The model under review builds one solid part; all positions refer to its coordinate system, in mm. A direction names the side the tool comes from. Coordinates: 2 decimals unless noted, no trailing zeros. Write each loop counter-clockwise with the first axis right and the second up, starting at its lowest first coordinate (ties: lowest second). Pieces come first, ordered by that corner, then holes.
1) Add section B-B, the plane x = 3. State the section outline as (y, z) points.
2) For P1, Ø1, axis at x = 7.5, y = -1.5, coming from the -Z side; P2, Ø4, axis at x = 22.5, z = -5, coming from the +Y side; P3, Ø0.6, axis at y = -1, z = -16, coming from the -X side, all flat-tipped, find the tip position at first contact; note any pin that passes through.
3) Add section A-A, the plane z = -14.5. State the section outline as (x, y) points, then the cut area to 3 significant figures.
4) Add section C-C, the plane y = 4.5. State the section outline as (x, z) points.
5) For line 1 (Y direction, x = 6, z = -8.75); line 2 (Y direction, x = 30.5, z = -13.5), list the stretches that pass through material, from the lowest coordinate up.
6) Add section D-D, the plane x = 28.5. State the section outline as (y, z) points.
7) Mouldability with a two-part tool opening along Z and no side actions: class faces 1 (the cylindrical face through (25.463, 8.951, -8.033)), 2 (the cylindrical face through (9.513, 0.507, -0.911)), 3 (the flat face through (16, 1, -13)) as released by +Z, released by -Z, zero draft, split by the parting line, or undercut.
8) Machinability: for faces 4 (the flat face through (13, -1, -22.429)), 5 (the flat face through (0.278, -1, -13)), 6 (the cylindrical face through (0.688, 0.507, -21.893)), which of the approach directions +Z, -Z, +X, -X, +Y, -Y give a long, thin tool a straight path to every point of the face, cutting with its end or side? Answer none if there is none.
from build123d import *

# Parameters (mm, degrees)
SKETCH1_W           = 33
SKETCH1_H           = 25
BOSS_EXTRUDE1_DEPTH = 1
CUT_EXTRUDE1_DEPTH  = 2
SKETCH3_R           = 0.4
SKETCH3_R_2         = 0.442084783
SKETCH3_R_3         = 0.458227678
CUT_EXTRUDE2_DEPTH  = 2
SKETCH4_R           = 0.75
BOSS_EXTRUDE2_DEPTH = 17
BOSS_EXTRUDE3_DEPTH = 2


with BuildPart() as part:
    # Sketch1 → Boss-Extrude1 (new body)
    with BuildSketch(Plane(origin=(0, 0, 0), x_dir=(1, 0, 0), z_dir=(0, 1, 0))):
        with Locations((16.5, 12.5)):
            Rectangle(SKETCH1_W, SKETCH1_H)
    extrude(amount=BOSS_EXTRUDE1_DEPTH)

    # Sketch2 → Cut-Extrude1 (cut, through all)
    with BuildSketch(Plane.XZ):
        Polygon((33, 0), (26.482981269, 0), (33, -7.837809095), align=None)
        Polygon((33, -17.162190905), (33, -25), (26.482981269, -25), align=None)
    extrude(amount=-CUT_EXTRUDE1_DEPTH, mode=Mode.SUBTRACT)

    # Sketch3 → Cut-Extrude2 (cut, through all)
    with BuildSketch(Plane(origin=(0, 1, 0), x_dir=(1, 0, 0), z_dir=(0, 1, 0))):
        with Locations((7.143852183, 23.936106005)):
            Circle(SKETCH3_R)
        with Locations((9.143852183, 23.936106005)):
            Circle(SKETCH3_R)
        with Locations((11.143852183, 23.936106005)):
            Circle(SKETCH3_R)
        with Locations((13.143852183, 23.936106005)):
            Circle(SKETCH3_R)
        with Locations((15.143852183, 23.936106005)):
            Circle(SKETCH3_R)
        with Locations((17.143852183, 23.936106005)):
            Circle(SKETCH3_R)
        with Locations((19.143852183, 23.936106005)):
            Circle(SKETCH3_R)
        with Locations((21.143852183, 23.936106005)):
            Circle(SKETCH3_R)
        with Locations((23.143852183, 23.936106005)):
            Circle(SKETCH3_R)
        with Locations((25.143852183, 23.936106005)):
            Circle(SKETCH3_R)
        with Locations((25.143852183, 1.063893995)):
            Circle(SKETCH3_R)
        with Locations((23.143852183, 1.063893995)):
            Circle(SKETCH3_R)
        with Locations((21.143852183, 1.063893995)):
            Circle(SKETCH3_R)
        with Locations((19.143852183, 1.063893995)):
            Circle(SKETCH3_R)
        with Locations((17.143852183, 1.063893995)):
            Circle(SKETCH3_R)
        with Locations((15.143852183, 1.063893995)):
            Circle(SKETCH3_R)
        with Locations((13.143852183, 1.063893995)):
            Circle(SKETCH3_R)
        with Locations((11.143852183, 1.063893995)):
            Circle(SKETCH3_R)
        with Locations((9.143852183, 1.063893995)):
            Circle(SKETCH3_R)
        with Locations((7.143852183, 1.063893995)):
            Circle(SKETCH3_R)
        with Locations((0.784299075, 22.325061426)):
            Circle(SKETCH3_R_2)
        with Locations((24.152709784, 2.722277331)):
            Circle(SKETCH3_R_3)
    extrude(amount=-CUT_EXTRUDE2_DEPTH, mode=Mode.SUBTRACT)

    # Sketch4 → Boss-Extrude2 (add)
    with BuildSketch(Plane(origin=(0, 1, 0), x_dir=(1, 0, 0), z_dir=(0, 1, 0))):
        with Locations((26.211922043, 8)):
            Circle(SKETCH4_R)
    extrude(amount=BOSS_EXTRUDE2_DEPTH)

    # Sketch5 → Revolve1 (revolve)
    with BuildSketch(Plane.XY.offset(-8)):
        with BuildLine():
            Line((26.211922043, 18), (26.211922043, 23))
            ThreePointArc((26.211922043, 23), (25.525593233, 22.727999503), (25.211922043, 22.059686783))
            Line((25.211922043, 22.059686783), (24.961922043, 18))
            ThreePointArc((24.961922043, 18), (25.081321038, 17.489279713), (25.461922043, 17.128399944))
            Line((25.461922043, 17.128399944), (25.461922043, 18))
            Line((25.461922043, 18), (26.211922043, 18))
        make_face()
    revolve(axis=Axis((26.211922043, 18, -8), (0, 1, 0)))

    # Sketch6 → Boss-Extrude3 (add)
    with BuildSketch(Plane.XZ):
        with BuildLine():
            Line((24.507853381, -22.428957603), (0.778175079, -22.428957603))
            ThreePointArc((0.778175079, -22.428957603), (0.424621688, -22.282510994), (0.278175079, -21.928957603))
            Line((0.278175079, -21.928957603), (0.278175079, -2.903294195))
            ThreePointArc((0.278175079, -2.903294195), (0.424621688, -2.549740805), (0.778175079, -2.403294195))
            Line((0.778175079, -2.403294195), (24.507853381, -2.403294195))
            ThreePointArc((24.507853381, -2.403294195), (24.861406772, -2.549740805), (25.007853381, -2.903294195))
            Line((25.007853381, -2.903294195), (25.007853381, -21.928957603))
            ThreePointArc((25.007853381, -21.928957603), (24.861406772, -22.282510994), (24.507853381, -22.428957603))
        make_face()
    extrude(amount=BOSS_EXTRUDE3_DEPTH)


solid = part.part
Geometry results:
1. outline: (-2, -22.43) - (0, -22.43) - (0, -25) - (1, -25) - (1, 0) - (0, 0) - (0, -2.4) - (-2, -2.4) - close
2. P1: stops at z = -22.43
2. P2: stops at y = 1
2. P3: stops at x = 0.28
3. outline: (0, 0) - (0.28, 0) - (0.28, -2) - (25.01, -2) - (25.01, 0) - (33, 0) - (33, 1) - (0, 1) - close
3. area: 82.5 mm2
4. outline: circle Ø1.5 at (26.21, -8)
5. line 1: y = -2 to 1
5. line 2: y = 0 to 1
6. outline: (0, -22.57) - (1, -22.57) - (1, -2.43) - (0, -2.43) - close
7. face 1: split by the parting line
7. face 2: undercut
7. face 3: zero draft
8. face 4: -Z, +X, -X, -Y
8. face 5: +Z, -Z, -X, -Y
8. face 6: +Y
